Can you work these out from the model? Positions are in its coordinate system, mm. A direction names the side the tool comes from. Coordinates: 2 decimals unless noted, no trailing zeros. Order: outer loops, then holes, each group sorted by start corner. A loop starts at its lowest first (then second) coordinate and runs counter-clockwise, first axis right, second up.
```python
from build123d import *

# Parameters (mm, degrees)
BOSS_EXTRUDE1_DEPTH = 3
SKETCH2_R           = 1.5
CUT_EXTRUDE1_DEPTH  = 3
BOSS_EXTRUDE2_START = 3
SKETCH3_R           = 1.5
BOSS_EXTRUDE2_DEPTH = 3


with BuildPart() as part:
    # Sketch1 → Boss-Extrude1 (new body)
    with BuildSketch(Plane(origin=(0, 0, 0), x_dir=(1, 0, 0), z_dir=(0, 1, 0))):
        Polygon((-22, 64), (-16.5, 0), (-10, 0), (-10, -6.5), (10, -6.5), (10, 0), (16.5, 0), (23.1, 64), (27.3, 64), (27.3, 108.3), (22, 108.3), (22, 111.6), (-22, 111.6), (-22, 108.3), (-27.3, 108.3), (-27.3, 64), align=None)
    extrude(amount=BOSS_EXTRUDE1_DEPTH)

    # Sketch2 → Cut-Extrude1 (cut)
    with BuildSketch(Plane.XZ):
        with Locations(Location((23.65, -102.1, 0), (0, 0, 270))):
            Circle(SKETCH2_R)
        with Locations(Location((-20.45, -102.1, 0), (0, 0, 270))):
            Circle(SKETCH2_R)
    extrude(amount=-CUT_EXTRUDE1_DEPTH, mode=Mode.SUBTRACT)

    # Sketch3 → Boss-Extrude2 (add)
    with BuildSketch(Plane.XZ.offset(BOSS_EXTRUDE2_START)):
        Polygon((-22, -64), (23.1, -64), (27.3, -64), (27.3, -108.3), (22, -108.3), (22, -111.6), (-22, -111.6), (-22, -108.3), (-27.3, -108.3), (-27.3, -64), align=None)
        with Locations(Location((-20.45, -102.1, 0), (0, 0, 270))):
            Circle(SKETCH3_R, mode=Mode.SUBTRACT)
        with Locations(Location((23.65, -102.1, 0), (0, 0, 270))):
            Circle(SKETCH3_R, mode=Mode.SUBTRACT)
    extrude(amount=-BOSS_EXTRUDE2_DEPTH)


solid = part.part
```
1. Imagine slicing it at B-B on z = -102.1. Please give me the cut outline in (x, y), then the cut area to 3 significant figures.
Completed:
outline: (-27.3, -3) - (-21.95, -3) - (-21.95, 3) - (-27.3, 3) - close; (-18.95, -3) - (22.15, -3) - (22.15, 3) - (-18.95, 3) - close; (25.15, -3) - (27.3, -3) - (27.3, 3) - (25.15, 3) - close
area: 292 mm2
2. Thinking about a two-plate mould opening in X: for faces 5 (the cylindrical face through (-20, -0.04, -103.53)), 6 (the flat face through (0, 0, -111.6)), 7 (the flat face through (-22, 0, -110)), 8 (the cylindrical face through (24.1, -0.04, -103.53)), which applies, pulls with the +X half, pulls with the -X half, needs draft (parallel to the pull), parting line crosses it, or undercut?
Completed:
face 5: undercut
face 6: needs draft
face 7: pulls with the -X half
face 8: undercut
3. Please list where these lines run through material, in increasing order: probe 1 along X at (y, z) = (0.75, -102.1); probe 2 along Z at (x, y) = (-2, -0.8); probe 3 along Z at (x, y) = (-11, 1.7).
Completed:
probe 1: x = -27.3 to -21.95, -18.95 to 22.15, 25.15 to 27.3
probe 2: z = -111.6 to -64
probe 3: z = -111.6 to 0
4. Imagine slicing it at D-D on x = 6.5. Please give me the cut outline in (y, z), then the cut area to 3 significant figures.
Completed:
outline: (-3, -111.6) - (3, -111.6) - (3, 6.5) - (0, 6.5) - (0, -64) - (-3, -64) - close
area: 497 mm2
5. I'm going to push flat-ended pins straight in: pin 1 (2.5 mm diameter, centred on x = -13.5, y = 1.5, fed in from +Z); pin 2 (10 mm diameter, centred on x = 8, z = -13, fed in from -Y); pin 3 (1 mm diameter, centred on y = 1.5, z = -12, fed in from +X); pin 4 (3.5 mm diameter, centred on y = -1, z = -109.5, fed in from +X). Where does each tip first touch, or does it pass through?
Completed:
pin 1: stops at z = 0
pin 2: stops at y = 0
pin 3: stops at x = 17.79
pin 4: stops at x = 27.3
6. On a 3-axis mill with a long thin cutter (end or side, diameter ignored), from which of +Z, -Z, +X, -X, +Y, -Y can I reach the whole of each face in a straight line? I mean faces 1 (the flat face through (-25, 0, -108.3)), 2 (the flat face through (25, 0, -108.3)), 3 (the flat face through (13, 1, 0)), 4 (the flat face through (-10, 1, 3)). Say none if no direction works.
Completed:
face 1: -Z, -X, +Y, -Y
face 2: -Z, +X, +Y, -Y
face 3: +Z, +X, +Y, -Y
face 4: +Z, -X, +Y, -Y
7. Imagine slicing it at C-C on x = -20.45. Please give me the cut outline in (y, z).
Completed:
outline: (-3, -111.6) - (3, -111.6) - (3, -103.6) - (-3, -103.6) - close; (-3, -100.6) - (3, -100.6) - (3, -45.96) - (0, -45.96) - (0, -64) - (-3, -64) - close
8. Imagine slicing it at A-A on y = -0.9. Please give me the cut outline in (x, z), then the cut area to 3 significant figures.
Completed:
outline: (-27.3, -108.3) - (-22, -108.3) - (-22, -111.6) - (22, -111.6) - (22, -108.3) - (27.3, -108.3) - (27.3, -64) - (-27.3, -64) - close; hole circle Ø3 at (-20.45, -102.1); hole circle Ø3 at (23.65, -102.1)
area: 2,550 mm2
